Geometry check sheet. Reference: drawing and pictorial views, mm from the part's lowest x, y, z. A direction names the side the tool comes from. Round coordinates to 2 decimals unless told otherwise and drop trailing zeros. Order: outer loops, then holes, each group sorted by start corner. A loop starts at its lowest first (then second) coordinate and runs counter-clockwise, first axis right, second up.
Q1. Cross-section at C-C on z = 21.5. Record the cut outline in (x, y), then the cut area to 3 significant figures.
Q2. Set-up check for the marked faces 1, 2 and 3: record each of +Z, -Z, +X, -X, +Y, -Y from which the full face is reachable in a straight line by a thin tool's end or side.
Q3. Cross-section at A-A on y = 12.7. Record the cut outline in (x, z), then the cut area to 3 significant figures.
Q4. Scan lines: probe 1 along X at (y, z) = (29, 29); probe 2 along Z at (x, y) = (37, 63.5). Record each from-to range of solid material in increasing order.
Q5. Cross-section at B-B on z = 12.7. Record the cut outline in (x, y).
Q6. Depth check by flat-ended pin: P1, Ø20.5, axis at y = 34, z = 41.5, coming from the +X side; P2, Ø12, axis at x = 40, y = 45.5, coming from the -Z side; P3, Ø12.5, axis at x = 8, z = 33.5, coming from the -Y side; P4, Ø20.5, axis at y = 7.5, z = 8.5, coming from the -X side. Enter the tip coordinate at first touch or a pass-through.
Q7. Cross-section at D-D on x = 43. Record the cut outline in (y, z), then the cut area to 3 significant figures.
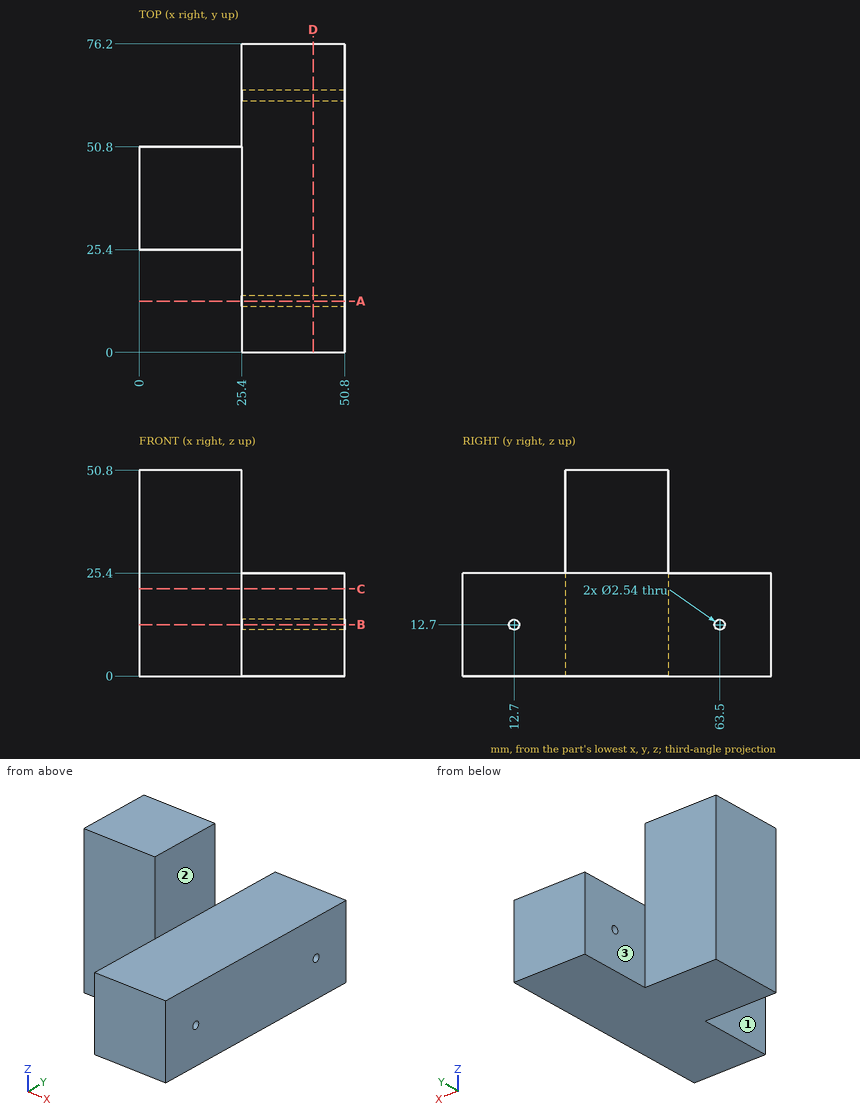
Results found:
1. outline: (0, 25.4) - (25.4, 25.4) - (25.4, 0) - (50.8, 0) - (50.8, 76.2) - (25.4, 76.2) - (25.4, 50.8) - (0, 50.8) - close
1. area: 2,580 mm2
2. face 1: +Z, -Z, -X, -Y
2. face 2: +Z, +X, +Y, -Y
2. face 3: +Z, -Z, -X, +Y
3. outline: (25.4, 0) - (50.8, 0) - (50.8, 11.43) - (25.4, 11.43) - close; (25.4, 13.97) - (50.8, 13.97) - (50.8, 25.4) - (25.4, 25.4) - close
3. area: 581 mm2
4. probe 1: x = 0 to 25.4
4. probe 2: z = 0 to 11.43, 13.97 to 25.4
5. outline: (0, 25.4) - (25.4, 25.4) - (25.4, 13.97) - (50.8, 13.97) - (50.8, 62.23) - (25.4, 62.23) - (25.4, 50.8) - (0, 50.8) - close; (25.4, 0) - (50.8, 0) - (50.8, 11.43) - (25.4, 11.43) - close; (25.4, 64.77) - (50.8, 64.77) - (50.8, 76.2) - (25.4, 76.2) - close
6. P1: stops at x = 25.4
6. P2: stops at z = 0
6. P3: stops at y = 25.4
6. P4: stops at x = 25.4
7. outline: (0, 0) - (76.2, 0) - (76.2, 25.4) - (0, 25.4) - close; hole circle Ø2.54 at (12.7, 12.7); hole circle Ø2.54 at (63.5, 12.7)
7. area: 1,930 mm2
